The listing builds one solid part. Answer for the finished solid, in the listing's coordinates (mm). Face numbers are marked on the shaded views. A direction names the side the tool comes from. Round coordinates to 2 decimals unless told otherwise and drop trailing zeros. Write each loop counter-clockwise with the first axis right and the second up, starting at its lowest first coordinate (ties: lowest second). Pieces come first, ordered by that corner, then holes. Notation, with made-up numbers: M 19,27 L 45,27 A18 ccw 45,53 Z; hole C 14,21.25 d9. An arc over 180 degrees is marked long. Write each question's results on one line, items separated by ' | '.
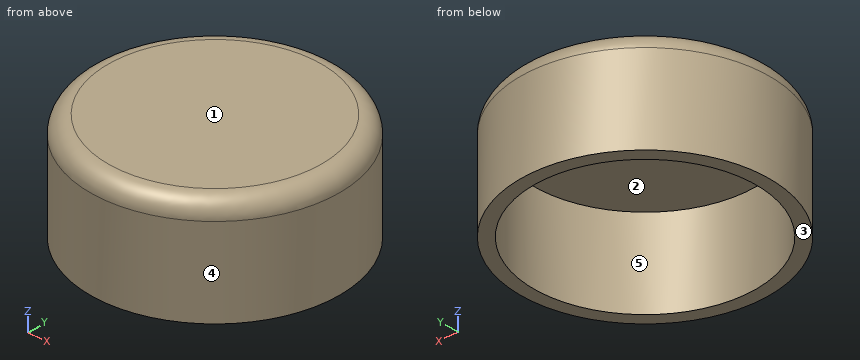
Autodesk Fusion 360 part; units mm, degrees
sketch "Sketch1" plane through (0, 0, 0) normal (0, 0, 1) x (1, 0, 0)
  circle A0 centre (0, 0) radius 14
  dimension "d1" = 28
extrude "Extrude1" add sketch "Sketch1" along normal blind 12
sketch "Sketch4" plane through (0, 0, 0) normal (0, 0, -1) x (1, 0, 0)
  circle A0 centre (0, 0) radius 14
  circle A1 centre (0, 0) radius 12.5
  dimension "d5" = 25
hole "Hole1" at (0, 0, 0) direction (0, 0, 1) diameter 25 depth 10 tip angle 180
thread "Thread1" thread offset 0 thread length 10
fillet "Fillet1" radius 2 1 edges at (-13.0526, -5.0626, 12)
1) Each of these flat-tipped pins is pushed along its axis until it touches: pin 1 (1 mm diameter, centred on x = 7, z = 8, fed in from +Y); pin 2 (2 mm diameter, centred on y = -5, z = 6, fed in from -X). Where does it stop, or does it pass through?
Return value:
pin 1: y = 12.4 | pin 2: x = -13.42
2) A tool of negligible diameter and unlimited length cuts with its end or side. For the marked faces 1 and 2, from which of +Z, -Z, +X, -X, +Y, -Y can it reach the whole face along a straight path? Write none if from no direction.
Return value:
face 1: +Z, +X, -X, +Y, -Y | face 2: -Z
3) Section A-A (x = 0) is taken. Determine the outline of the cut face in (y, z), then the cut area to 3 significant figures.
Return value:
outline: M -14,0 L -12.5,0 L -12.5,10 L 12.5,10 L 12.5,0 L 14,0 L 14,10 A2 ccw 12,12 L -12,12 A2 ccw -14,10 Z | area: 84.3 mm²
4) The mould has two halves that part along Y. Classify the marked faces 3, 4 and 5: +Y half, -Y half, draft (parallel to the pull), parting line (faces both ways), or undercut.
Return value:
face 3: draft | face 4: parting line | face 5: undercut
5) Find the intervals of material crossed by line 1 (Y direction, x = 0, z = 4.25); line 2 (Z direction, x = 1, y = -10.75); line 3 (X direction, y = 3.25, z = 4.5), in increasing order.
Return value:
line 1: -14 to -12.5, 12.5 to 14 | line 2: 10 to 12 | line 3: -13.62 to -12.07, 12.07 to 13.62
6) Section C-C (z = 8.75) is taken. Determine the outline of the cut face in (x, y), then the cut area to 3 significant figures.
Return value:
outline: C 0,0 d28; hole C 0,0 d25 | area: 125 mm²
